For this review, take the finished solid that the model builds, in its own axes (mm). A direction names the side the tool comes from. Give positions to 0.01 mm unless a question says otherwise; leave off trailing zeros. Order: outer loops, then holes, each group sorted by start corner. A loop starts at its lowest first (then second) coordinate and runs counter-clockwise, first axis right, second up. Notation, with made-up numbers: M 32.25,-19.75 L 75.25,-19.75 A38 cw 75.25,19.25 Z; hole C 48,67.5 d4. An arc over 180 degrees is marked long. Use CSV: the item, a comma, the result in double quotes. Start each with the question number.
(1) Consider section B-B (x = -3.5). Write out the cut boundary in (y, z), and give its area (3 significant figures).
(2) Consider section C-C (y = 1.75). Write out the cut boundary in (x, z), and give its area (3 significant figures).
(3) Consider section A-A (z = -22.75). Write out the cut boundary in (x, y).
(4) Consider section D-D (z = -30.5). Write out the cut boundary in (x, y), and give its area (3 significant figures).
(5) Clearance check with flat-ended pins moving along their axes: P1, Ø1.7, axis at x = 1.5, y = -1, coming from the -Z side; P2, Ø3, axis at x = -1, y = 0, coming from the +Z side. State where each tip first meets the part, or that it passes through.
(6) Tool access review of faces 1 (the face through (-0.506, -3.997, -31.632)), 2 (the face through (0, 2.79, -21)), 3 (the face through (2.62, 1.54, -44.11)), 4 (the face through (-0.98, 4.39, -31.12)): name each direction out of +Z, -Z, +X, -X, +Y, -Y from which nothing blocks a thin tool from reaching the whole face with its end or side.
(7) Wall thickness on L1, parallel to Z at x = 1.25, y = 2; L2, parallel to Y at x = -1, z = -22.75; L3, parallel to Y at x = 2.5, z = -23.5: over which ranges is each line inside the solid? List them lowest first. Write a range as from..to.
(8) Draft analysis for pull direction Z (two halves, no side actions). For faces 5 (the face through (0, -2.79, -41)), 6 (the face through (3, 2, -17.5)), 7 (the face through (0.01, -4.01, -31.61)), state which applies: pulls with the +Z half, pulls with the -Z half, needs draft (parallel to the pull), parting line crosses it, or undercut.
```python
from build123d import *

# Parameters (mm, degrees)
SKETCH1_W          = 4.5
SKETCH1_H          = 26.85997733
CUT_EXTRUDE1_DEPTH = 7
CUT_EXTRUDE2_DEPTH = 7
CHAMFER1_SIZE      = 0.5
CUT_EXTRUDE3_DEPTH = 1


with BuildPart() as part:
    # Sketch1 → Revolve-Thin1 (revolve)
    with BuildSketch(Plane(origin=(0, 0, 0), x_dir=(1, 0, 0), z_dir=(0, 1, 0))):
        with Locations((2.25, 30.929988665)):
            Rectangle(SKETCH1_W, SKETCH1_H)
    revolve(axis=Axis((0, 0, 0), (0, 0, -1)))

    # Sketch2 → Cut-Extrude1 (cut)
    with BuildSketch(Plane.XY.offset(-17.5)):
        Polygon((1.610807251, 2.79), (-1.610807251, 2.79), (-3.221614502, 0), (-1.610807251, -2.79), (1.610807251, -2.79), (3.221614502, 0), align=None)
    extrude(amount=-CUT_EXTRUDE1_DEPTH, mode=Mode.SUBTRACT)

    # Sketch3 → Cut-Extrude2 (cut)
    with BuildSketch(Plane(origin=(0, 0, -44.35997733), x_dir=(-1, 0, 0), z_dir=(0, 0, -1))):
        Polygon((1.610807251, 2.79), (-1.610807251, 2.79), (-3.221614502, 0), (-1.610807251, -2.79), (1.610807251, -2.79), (3.221614502, 0), align=None)
    extrude(amount=-CUT_EXTRUDE2_DEPTH, mode=Mode.SUBTRACT)

    # Chamfer1
    chamfer1_edges = [part.edges().sort_by_distance(p)[0] for p in [
        (2.416210877, 1.395, -17.5),
        (0, 2.79, -17.5),
        (-2.416210877, 1.395, -17.5),
        (-2.416210877, -1.395, -17.5),
        (0, -2.79, -17.5),
        (2.416210877, -1.395, -17.5),
        (-2.416210877, 1.395, -44.35997733),
        (0, 2.79, -44.35997733),
        (2.416210877, 1.395, -44.35997733),
        (2.416210877, -1.395, -44.35997733),
        (0, -2.79, -44.35997733),
        (-2.416210877, -1.395, -44.35997733),
    ]]
    chamfer(chamfer1_edges, length=CHAMFER1_SIZE)

    # Sketch4 → Cut-Extrude3 (cut)
    with BuildSketch(Plane(origin=(0, -4.5, 0), x_dir=(1, 0, 0), z_dir=(0, 1, 0))):
        with BuildLine():
            Line((-0.735236378, 34.104988665), (-0.183809095, 34.104988665))
            add(Edge.make_bspline(
                [(-0.183809095, 34.104988665), (-0.142887229, 34.104821435), (-0.063984952, 34.104498996), (0.049479088, 34.099913909), (0.153619775, 34.092996425), (0.248313279, 34.083867435), (0.333638661, 34.071201473), (0.40941848, 34.055993448), (0.47613676, 34.039057193), (0.516147477, 34.02331892), (0.534890825, 34.015946197)],
                knots=[0, 0, 0, 0, 0.000122758, 0.000236692, 0.000340599, 0.000435844, 0.000522015, 0.000599225, 0.000667726, 0.000728098, 0.000728098, 0.000728098, 0.000728098], degree=3))
            add(Edge.make_bspline(
                [(0.534890825, 34.015946197), (0.555993425, 34.006429933), (0.597245667, 33.987827142), (0.656357727, 33.95629427), (0.711711569, 33.922324809), (0.762389804, 33.884637999), (0.8094619, 33.84482071), (0.852635966, 33.802494227), (0.891564361, 33.757008969), (0.926655631, 33.709180776), (0.957858636, 33.659071505), (0.984643202, 33.606434054), (1.007803352, 33.551714066), (1.025889509, 33.49431609), (1.04092128, 33.434929127), (1.050643284, 33.373178483), (1.057485172, 33.309272455), (1.058047365, 33.265888615), (1.058333333, 33.243820796)],
                knots=[0, 0, 0, 0, 6.9431e-05, 0.000135726, 0.000200852, 0.000264074, 0.000324989, 0.000385705, 0.00044524, 0.000504393, 0.000563519, 0.000622115, 0.000681412, 0.000741551, 0.000802483, 0.00086501, 0.000928929, 0.000995103, 0.000995103, 0.000995103, 0.000995103], degree=3))
            add(Edge.make_bspline(
                [(1.058333333, 33.243820796), (1.057660809, 33.216664827), (1.056333136, 33.163054546), (1.047657842, 33.083998974), (1.031477343, 33.008136947), (1.009687089, 32.93522949), (0.982690716, 32.864804536), (0.947875359, 32.798087533), (0.907633136, 32.733916018), (0.861157476, 32.67313132), (0.809209736, 32.61517584), (0.749228296, 32.563460322), (0.684531415, 32.51450675), (0.612461254, 32.471597247), (0.53499992, 32.431738139), (0.45038063, 32.397967081), (0.360191554, 32.366801607), (0.296952619, 32.351203721), (0.264583333, 32.343219835)],
                knots=[0, 0, 0, 0, 8.1472e-05, 0.00016084, 0.000238178, 0.00031384, 0.000388957, 0.000464053, 0.000539224, 0.00061593, 0.000693367, 0.000772226, 0.000853128, 0.000936463, 0.001023502, 0.00111421, 0.001209545, 0.001309511, 0.001309511, 0.001309511, 0.001309511], degree=3))
            Line((0.264583333, 32.343219835), (0.997275641, 30.929988665))
            Line((0.997275641, 30.929988665), (0.360621995, 30.929988665))
            Line((0.360621995, 30.929988665), (-0.356805889, 32.313963024))
            Line((-0.356805889, 32.313963024), (-0.41023137, 32.313963024))
            Line((-0.41023137, 32.313963024), (-0.605488782, 30.929988665))
            Line((-0.605488782, 30.929988665), (-1.180448718, 30.929988665))
            Line((-1.180448718, 30.929988665), (-0.735236378, 34.104988665))
        make_face()
        with BuildLine():
            add(Edge.make_bspline(
                [(-0.335817308, 32.843129691), (-0.294894066, 32.843508532), (-0.2166182, 32.84423316), (-0.104827079, 32.849303715), (-0.004219131, 32.857224722), (0.08509361, 32.868749131), (0.16339231, 32.882182886), (0.230523904, 32.899038904), (0.286593934, 32.919072013), (0.332485643, 32.942831056), (0.369661123, 32.970726112), (0.40183809, 33.00049459), (0.428631207, 33.033817084), (0.450737928, 33.070134204), (0.467788114, 33.109521218), (0.480083934, 33.152244969), (0.486882391, 33.198020591), (0.487927508, 33.229595041), (0.488461538, 33.245728849)],
                knots=[0, 0, 0, 0, 0.000122766, 0.000234821, 0.000335651, 0.000425427, 0.000504898, 0.000573853, 0.000632811, 0.000683169, 0.0007282, 0.000771845, 0.000814359, 0.000856026, 0.000899036, 0.000942718, 0.000989043, 0.001037447, 0.001037447, 0.001037447, 0.001037447], degree=3))
            add(Edge.make_bspline(
                [(0.488461538, 33.245728849), (0.487770257, 33.264022258), (0.486429265, 33.299508964), (0.474830234, 33.35062006), (0.454996287, 33.39698474), (0.427122393, 33.438159863), (0.392337213, 33.474465682), (0.349901429, 33.504369125), (0.300298842, 33.527903238), (0.253836196, 33.543471254), (0.210053836, 33.552396101), (0.169082237, 33.558639509), (0.120514754, 33.564294057), (0.064292994, 33.568668304), (0.000652546, 33.571550346), (-0.070576621, 33.574306307), (-0.149461846, 33.575296954), (-0.204585812, 33.575641686), (-0.23341847, 33.575821998)],
                knots=[0, 0, 0, 0, 5.483e-05, 0.000106364, 0.000156221, 0.00020526, 0.000254739, 0.000306272, 0.000360034, 0.000418964, 0.000452769, 0.000493968, 0.000543275, 0.000599421, 0.000663102, 0.000734382, 0.000813258, 0.000899759, 0.000899759, 0.000899759, 0.000899759], degree=3))
            Line((-0.23341847, 33.575821998), (-0.335817308, 32.843129691))
        make_face(mode=Mode.SUBTRACT)
    extrude(amount=CUT_EXTRUDE3_DEPTH, mode=Mode.SUBTRACT)


solid = part.part
```
Check result:
1,outline,"M -2.83,-44.36 L -0.52,-44.36 L 0,-44.1 L 0.52,-44.36 L 2.83,-44.36 L 2.83,-17.5 L 0.52,-17.5 L 0,-17.76 L -0.52,-17.5 L -2.83,-17.5 Z"
1,area,"152 mm^2"
2,outline,"M -4.15,-44.36 L -2.79,-44.36 L -2.21,-43.86 L -2.21,-37.36 L 2.21,-37.36 L 2.21,-43.86 L 2.79,-44.36 L 4.15,-44.36 L 4.15,-17.5 L 2.79,-17.5 L 2.21,-18 L 2.21,-24.5 L -2.21,-24.5 L -2.21,-18 L -2.79,-17.5 L -4.15,-17.5 Z"
2,area,"160 mm^2"
3,outline,"C 0,0 d9; hole M -3.22,0 L -1.61,-2.79 L 1.61,-2.79 L 3.22,0 L 1.61,2.79 L -1.61,2.79 Z"
4,outline,"C 0,0 d9"
4,area,"63.6 mm^2"
5,P1,"stops at z = -37.36"
5,P2,"stops at z = -24.5"
6,face 1,"-Y"
6,face 2,"+Z"
6,face 3,"-Z"
6,face 4,"+Z, -Z"
7,L1,"z = -37.36..-24.5"
7,L2,"y = -4.39..-2.79, 2.79..4.39"
7,L3,"y = -3.74..-1.25, 1.25..3.74"
8,face 5,"needs draft"
8,face 6,"pulls with the +Z half"
8,face 7,"undercut"
